from build123d import *

# Parameters (mm, degrees)
SKETCH1_W           = 44
SKETCH1_H           = 10
BOSS_EXTRUDE1_DEPTH = 8
SKETCH4_W           = 10
SKETCH4_H           = 10
BOSS_EXTRUDE2_DEPTH = 8
SKETCH3_R           = 1.6
CUT_EXTRUDE2_DEPTH  = 48.874836814
SKETCH5_W           = 10
SKETCH5_H           = 8
BOSS_EXTRUDE3_DEPTH = 10
SKETCH6_R           = 1.45
CUT_EXTRUDE3_DEPTH  = 49.989794856
FILLET2_R           = 2.5
FILLET1_R           = 3


with BuildPart() as part:
    # Sketch1 → Boss-Extrude1 (new body)
    with BuildSketch(Plane.XY):
        with Locations((22, -5)):
            Rectangle(SKETCH1_W, SKETCH1_H)
    extrude(amount=BOSS_EXTRUDE1_DEPTH)

    # Sketch4 → Boss-Extrude2 (add)
    with BuildSketch(Plane(origin=(0, 0, 0), x_dir=(-1, 0, 0), z_dir=(0, 0, -1))):
        with Locations((-5, -5)):
            Rectangle(SKETCH4_W, SKETCH4_H)
        with Locations((-39, -5)):
            Rectangle(SKETCH4_W, SKETCH4_H)
    extrude(amount=BOSS_EXTRUDE2_DEPTH)

    # Sketch3 → Cut-Extrude2 (cut, through all)
    with BuildSketch(Plane.XY.offset(8)):
        with Locations((18, -5)):
            Circle(SKETCH3_R)
        with Locations((26, -5)):
            Circle(SKETCH3_R)
    extrude(amount=-CUT_EXTRUDE2_DEPTH, mode=Mode.SUBTRACT)

    # Sketch5 → Boss-Extrude3 (add)
    with BuildSketch(Plane(origin=(0, -10, 0), x_dir=(-1, 0, 0), z_dir=(0, -1, 0))):
        with Locations((-5, 4)):
            Rectangle(SKETCH5_W, SKETCH5_H)
        with Locations((-39, 4)):
            Rectangle(SKETCH5_W, SKETCH5_H)
    extrude(amount=BOSS_EXTRUDE3_DEPTH)

    # Sketch6 → Cut-Extrude3 (cut, through all)
    with BuildSketch(Plane.XY):
        with Locations((5, -16)):
            Circle(SKETCH6_R)
        with Locations((39, -16)):
            Circle(SKETCH6_R)
    extrude(amount=-CUT_EXTRUDE3_DEPTH, mode=Mode.SUBTRACT)

    # Fillet2
    fillet2_edges = [part.edges().sort_by_distance(p)[0] for p in [
        (10, -20, -4),
        (0, -20, -4),
        (34, -20, -4),
        (44, -20, -4),
    ]]
    fillet(fillet2_edges, radius=FILLET2_R)

    # Fillet1
    fillet1_edges = [part.edges().sort_by_distance(p)[0] for p in [
        (0, 0, 0),
        (44, 0, 0),
        (44, -10, 4),
        (0, -10, 4),
    ]]
    fillet(fillet1_edges, radius=FILLET1_R)


solid = part.part
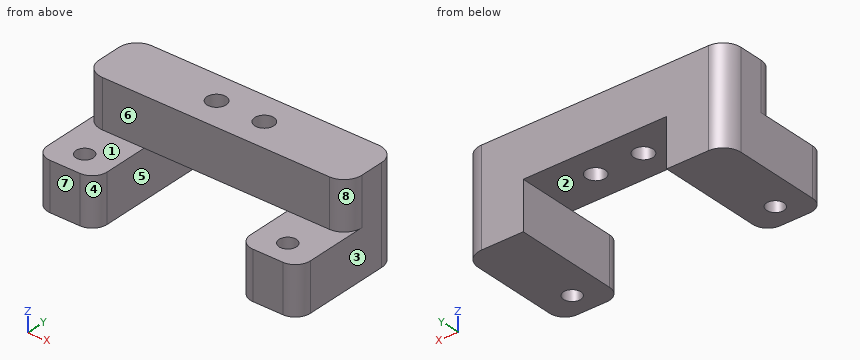
Work out the finished part from the listing and answer in its coordinate system (mm). Face numbers are marked on the shaded views. A direction names the side the tool comes from. Coordinates: 2 decimals unless noted, no trailing zeros. Loops run counter-clockwise (first coordinate to the right, second up) from the corner with the lowest first, then second, coordinate; pieces in that order, holes last. Notation, with made-up numbers: M -23,-27 L 28,-27 A33 ccw 28,5 Z; hole C 58,59.5 d11. An arc over 180 degrees is marked long. Answer in a Markdown table with one row per item. Add a question column.
1. Find section A-A, the plane z = -0.75. Write down the section's boundary in (x, y).
2. Find section C-C, the plane y = -5. Write down the section's boundary in (x, z), then the cut area to 3 significant figures.
3. Consider L1, parallel to Y at x = 39, z = -6.75; L2, parallel to X at y = -17.5, z = -5; L3, parallel to X at y = -17, z = -2.75. Determine where each line is inside the solid, lowest interval first.
4. A tool of negligible diameter and unlimited length cuts with its end or side. For the marked faces 5, 6, 7 and 8, from which of +Z, -Z, +X, -X, +Y, -Y can it reach the whole face along a straight path? Write none if from no direction.
5. Flat-ended cylindrical pins translate along their axes: P1, Ø6.5, axis at x = 31.5, z = 3.5, coming from the -Y side; P2, Ø5, axis at x = 37, y = -15, coming from the +Z side; P3, Ø5, axis at x = 27.5, y = -6.5, coming from the -Z side. Find the tip coordinate at first contact, or state that the pin passes through.
6. Find section D-D, the plane y = -11.75. Write down the section's boundary in (x, z).
7. The mould has two halves that part along X. Classify the marked faces 1, 2, 3 and 4: pulls with the +X half, pulls with the -X half, needs draft (parallel to the pull), parting line crosses it, or undercut.
8. Find section B-B, the plane x = 39. Write down the section's boundary in (y, z).
Reported:
| question | item | result |
|---|---|---|
| 1 | outline | M 0,-17.5 A2.5 ccw 2.5,-20 L 7.5,-20 A2.5 ccw 10,-17.5 L 10,0 L 3,0 A3 ccw 0,-3 Z; M 34,-17.5 A2.5 ccw 36.5,-20 L 41.5,-20 A2.5 ccw 44,-17.5 L 44,-3 A3 ccw 41,0 L 34,0 Z; hole C 5,-16 d2.9; hole C 39,-16 d2.9 |
| 2 | outline | M 0,-8 L 10,-8 L 10,0 L 16.4,0 L 16.4,8 L 0,8 Z; M 19.6,0 L 24.4,0 L 24.4,8 L 19.6,8 Z; M 27.6,0 L 34,0 L 34,-8 L 44,-8 L 44,8 L 27.6,8 Z |
| 2 | area | 461 mm^2 |
| 3 | L1 | y = -20 to -17.45, -14.55 to 0 |
| 3 | L2 | x = 0 to 10, 34 to 44 |
| 3 | L3 | x = 0 to 3.95, 6.05 to 10, 34 to 37.95, 40.05 to 44 |
| 4 | face 5 | -Z, +Y, -Y |
| 4 | face 6 | +Z, +X, -X, -Y |
| 4 | face 7 | +Z, -Z, +X, -X, -Y |
| 4 | face 8 | +Z, +X, -Y |
| 5 | P1 | stops at y = -10 |
| 5 | P2 | stops at z = 0 |
| 5 | P3 | stops at z = 0 |
| 6 | outline | M 0,-8 L 10,-8 L 10,0 L 0,0 Z; M 34,-8 L 44,-8 L 44,0 L 34,0 Z |
| 7 | face 1 | needs draft |
| 7 | face 2 | undercut |
| 7 | face 3 | pulls with the +X half |
| 7 | face 4 | undercut |
| 8 | outline | M -20,-8 L -17.45,-8 L -17.45,0 L -20,0 Z; M -14.55,-8 L 0,-8 L 0,8 L -10,8 L -10,0 L -14.55,0 Z |
